```python
from build123d import *

# Parameters (mm, degrees)
BOSS_EXTRUDE1_DEPTH = 10
SKETCH3_R           = 1.5
CUT_EXTRUDE1_DEPTH  = 39.487010796
SKETCH4_R           = 1.5
CUT_EXTRUDE2_DEPTH  = 39.487010796
SKETCH5_R           = 2.5
CUT_EXTRUDE3_DEPTH  = 10
SKETCH9_R           = 1.5
CUT_EXTRUDE4_DEPTH  = 37.742346142


with BuildPart() as part:
    # Sketch1 → Boss-Extrude1 (new body)
    with BuildSketch(Plane(origin=(0, 0, 0), x_dir=(1, 0, 0), z_dir=(0, 1, 0))):
        Polygon((-2.5, 12.5), (-2.5, 25), (-25, 25), (-25, 2.5), (-12.5, 2.5), (-12.5, -2.5), (-25, -2.5), (-25, -25), (-2.5, -25), (-2.5, -12.5), (2.5, -12.5), (2.5, -25), (25, -25), (25, -2.5), (12.5, -2.5), (12.5, 2.5), (25, 2.5), (25, 25), (2.5, 25), (2.5, 12.5), align=None)
    extrude(amount=BOSS_EXTRUDE1_DEPTH)

    # Sketch3 → Cut-Extrude1 (cut, symmetric)
    with BuildSketch(Plane.ZY.offset(2.5)):
        with Locations((-18.75, 5)):
            Circle(SKETCH3_R)
    cut_extrude1 = extrude(amount=CUT_EXTRUDE1_DEPTH, both=True, mode=Mode.SUBTRACT)

    # Mirror1: Cut-Extrude1 across plane
    add(cut_extrude1.mirror(Plane.XY), mode=Mode.SUBTRACT)

    # Sketch4 → Cut-Extrude2 (cut, symmetric)
    with BuildSketch(Plane.XY.offset(2.5)):
        with Locations(Location((-18.75, 5, 0), (0, 0, 270))):
            Circle(SKETCH4_R)
    cut_extrude2 = extrude(amount=CUT_EXTRUDE2_DEPTH, both=True, mode=Mode.SUBTRACT)

    # Mirror2: Cut-Extrude2 across plane
    add(cut_extrude2.mirror(Plane(origin=(0, 0, 0), x_dir=(0, 0, 1), z_dir=(1, 0, 0))), mode=Mode.SUBTRACT)

    # Sketch5 → Cut-Extrude3 (cut)
    with BuildSketch(Plane(origin=(0, 10, 0), x_dir=(1, 0, 0), z_dir=(0, 1, 0))):
        with Locations(Location((0, 0, 0), (0, 0, 270))):
            Circle(SKETCH5_R)
    extrude(amount=-CUT_EXTRUDE3_DEPTH, mode=Mode.SUBTRACT)

    # Sketch9 → Cut-Extrude4 (cut, through all)
    with BuildSketch(Plane(origin=(0, 10, 0), x_dir=(1, 0, 0), z_dir=(0, 1, 0))):
        with Locations(Location((-18.75, 18.75, 0), (0, 0, 270))):
            Circle(SKETCH9_R)
        with Locations(Location((18.75, 18.75, 0), (0, 0, 270))):
            Circle(SKETCH9_R)
        with Locations(Location((18.75, -18.75, 0), (0, 0, 270))):
            Circle(SKETCH9_R)
        with Locations(Location((-18.75, -18.75, 0), (0, 0, 270))):
            Circle(SKETCH9_R)
    extrude(amount=-CUT_EXTRUDE4_DEPTH, mode=Mode.SUBTRACT)


solid = part.part
```
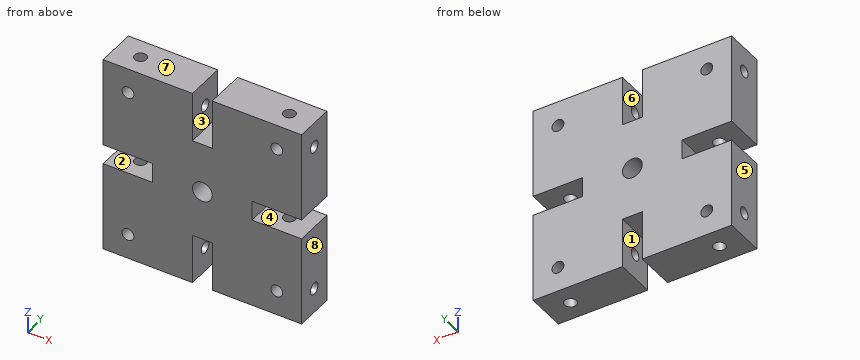
The listing builds one solid part. Answer for the finished solid, in the listing's coordinates (mm). Face numbers are marked on the shaded views. A direction names the side the tool comes from. Round coordinates to 2 decimals unless told otherwise and drop trailing zeros. Write each loop counter-clockwise with the first axis right and the second up, starting at its lowest first coordinate (ties: lowest second). Pieces come first, ordered by that corner, then holes. Notation, with made-up numbers: (23, 64.5) -> (44, 64.5) arc R11 ccw to (44, 80.5) -> close; hole circle Ø2 at (8, 84.5). An arc over 180 degrees is marked (long way). Write item = value, one per line.
1) For a pull along X with two mould halves and no side action, classify the marked faces 5, 6, 7 and 8 as released by +X, released by -X, zero draft, split by the parting line, or undercut.
Check values:
face_5 = released by -X
face_6 = undercut
face_7 = zero draft
face_8 = released by +X
2) Given pin 1 (1.5 mm diameter, centred on x = -1, y = 5, fed in from -Z); pin 2 (5 mm diameter, centred on x = -1, z = 11, fed in from -Y); pin 3 (1.5 mm diameter, centred on y = 4, z = 1, fed in from +X), each flat-ended and moving along its own axis, determine where each tip first touches the part or whether it passes through.
Check values:
pin_1 = -12.5
pin_2 = 0
pin_3 = 12.5
3) Section B-B on z = 13.5 is taken. Write down the section's boundary in (x, y).
Check values:
outline = (-25, 0) -> (-2.5, 0) -> (-2.5, 10) -> (-25, 10) -> close; (2.5, 0) -> (25, 0) -> (25, 10) -> (2.5, 10) -> close; hole circle Ø3 at (-18.75, 5); hole circle Ø3 at (18.75, 5)
4) Section D-D on x = -18.75 is taken. Give the number of separate pieces and of enclosed holes in the cut face, plus the area to 3 significant figures.
Check values:
separate_pieces = 8
enclosed_holes = 0
area = 273 mm²
5) Which of the six approach directions +Z, -Z, +X, -X, +Y, -Y give full straight-line access (tool end or side, diameter ignored) to the marked faces 1, 2, 3 and 4?
Check values:
face_1 = -Z, +Y, -Y
face_2 = -X, +Y, -Y
face_3 = +Z, +Y, -Y
face_4 = +X, +Y, -Y
6) Straight lines are drawn through the part: line 1 along Z through (x, y) = (22.9, 5); line 2 along Z through (x, y) = (22, 2.75). For each, find the intervals that lie inside material, in ascending order. Write a range as [from, to].
Check values:
line_1 = [-25, -20.25], [-17.25, -2.5], [2.5, 17.25], [20.25, 25]
line_2 = [-25, -2.5], [2.5, 25]
7) Section C-C on y = 8 is taken. Write down the section's boundary in (x, z), plus the area to 3 significant figures.
Check values:
outline = (-25, -25) -> (-2.5, -25) -> (-2.5, -12.5) -> (2.5, -12.5) -> (2.5, -25) -> (25, -25) -> (25, -2.5) -> (12.5, -2.5) -> (12.5, 2.5) -> (25, 2.5) -> (25, 25) -> (2.5, 25) -> (2.5, 12.5) -> (-2.5, 12.5) -> (-2.5, 25) -> (-25, 25) -> (-25, 2.5) -> (-12.5, 2.5) -> (-12.5, -2.5) -> (-25, -2.5) -> close; hole circle Ø3 at (-18.75, -18.75); hole circle Ø3 at (-18.75, 18.75); hole circle Ø5 at (0, 0); hole circle Ø3 at (18.75, -18.75); hole circle Ø3 at (18.75, 18.75)
area = 2,200 mm²
8) Section A-A on x = 14.5 is taken. Write down the section's boundary in (y, z), plus the area to 3 significant figures.
Check values:
outline = (0, -25) -> (10, -25) -> (10, -2.5) -> (0, -2.5) -> close; (0, 2.5) -> (10, 2.5) -> (10, 25) -> (0, 25) -> close; hole circle Ø3 at (5, -18.75); hole circle Ø3 at (5, 18.75)
area = 436 mm²
